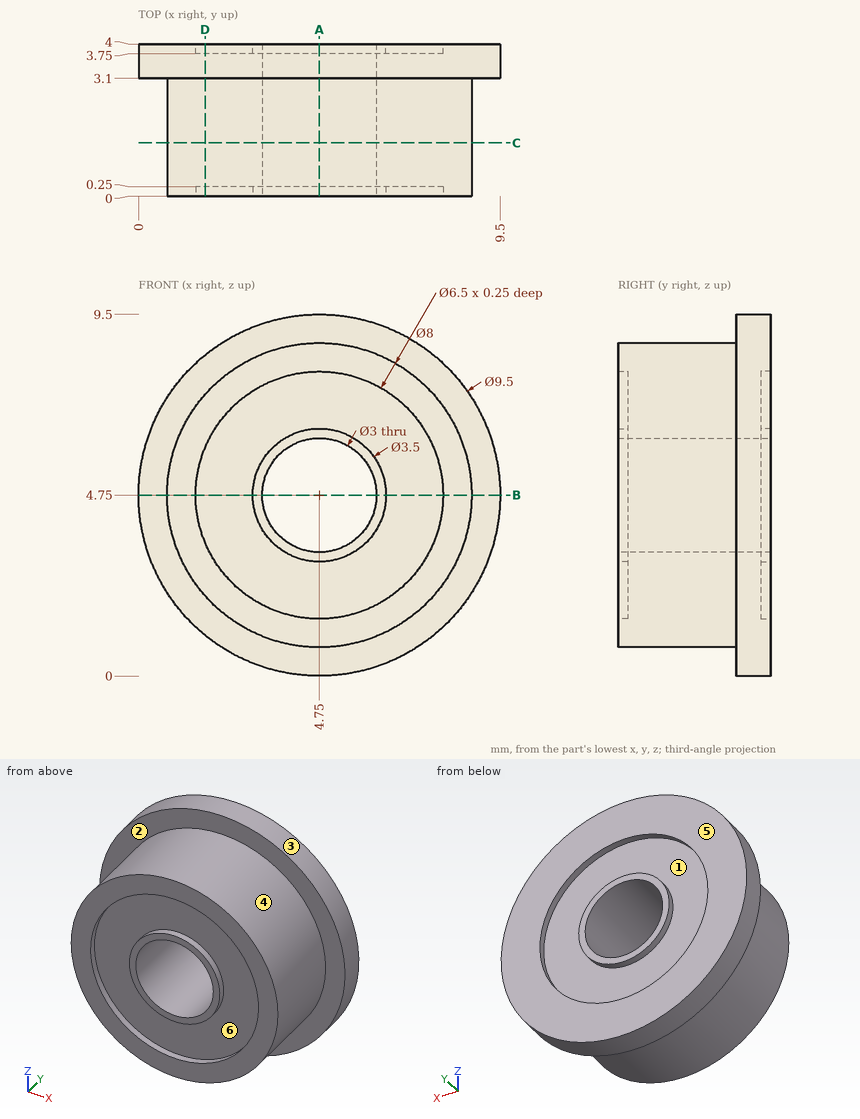
Print and shaded views of the part. All mm, measured from the part's lowest x, y and z. A direction names the side the tool comes from. Give positions to 0.01 mm unless a question says otherwise; leave off trailing zeros. Write each loop counter-clockwise with the first axis right and the second up, starting at its lowest first coordinate (ties: lowest second). Pieces come first, ordered by that corner, then holes. Notation, with made-up numbers: (36, -33.75) -> (62, -33.75) arc R24 ccw to (62, -20.75) -> close; hole circle Ø7 at (6.5, -30.75). An arc over 180 degrees is marked (long way). Use CSV: the item, a comma, the result in double quotes. Start each with the question number.
1) Cut at A-A on x = 4.75. List the corners of the cut face in (y, z), plus the area to 4 significant figures.
2) Drill centre lines: L1, parallel to X at y = 3.9, z = 4.75; L2, parallel to X at y = 0.15, z = 4.75; L3, parallel to X at y = 1.85, z = 4.75. Where is each one in solid material? Low to high.
3) Tool access for the marked faces 1, 2 and 3: list every direction of +Z, -Z, +X, -X, +Y, -Y with a clear straight run to the whole face (end or side of a thin tool).
4) Cut at D-D on x = 1.75. List the corners of the cut face in (y, z).
5) Cut at B-B on z = 4.75. List the corners of the cut face in (x, y), plus the area to 4 significant figures.
6) Cut at C-C on y = 1.4. List the corners of the cut face in (x, z).
7) Two-plate mould, pull along X, no slides. Class the marked faces 4, 5 and 6: released by +X, released by -X, zero draft, split by the parting line, or undercut.
8) Pin check, flat tips, straight feed: P1, Ø5, axis at x = 7.5, z = 5, coming from the -Y side; P2, Ø1.8, axis at x = 4.75, z = 4.75, coming from the -Y side. Stop position of each tip, or through.
Final values:
1,outline,"(0, 0.75) -> (3.1, 0.75) -> (3.1, 0) -> (4, 0) -> (4, 1.5) -> (3.75, 1.5) -> (3.75, 3) -> (4, 3) -> (4, 3.25) -> (0, 3.25) -> (0, 3) -> (0.25, 3) -> (0.25, 1.5) -> (0, 1.5) -> close; (0, 6.25) -> (4, 6.25) -> (4, 6.5) -> (3.75, 6.5) -> (3.75, 8) -> (4, 8) -> (4, 9.5) -> (3.1, 9.5) -> (3.1, 8.75) -> (0, 8.75) -> (0, 8) -> (0.25, 8) -> (0.25, 6.5) -> (0, 6.5) -> close"
1,area,"19.85 mm2"
2,L1,"x = 0 to 1.5, 3 to 3.25, 6.25 to 6.5, 8 to 9.5"
2,L2,"x = 0.75 to 1.5, 3 to 3.25, 6.25 to 6.5, 8 to 8.75"
2,L3,"x = 0.75 to 3.25, 6.25 to 8.75"
3,face 1,"+Y"
3,face 2,"-Y"
3,face 3,"+Y, -Y"
4,outline,"(0, 2.1) -> (3.1, 2.1) -> (3.1, 1.07) -> (4, 1.07) -> (4, 3.5) -> (3.75, 3.5) -> (3.75, 6) -> (4, 6) -> (4, 8.43) -> (3.1, 8.43) -> (3.1, 7.4) -> (0, 7.4) -> (0, 6) -> (0.25, 6) -> (0.25, 3.5) -> (0, 3.5) -> close"
5,outline,"(0, 3.1) -> (0.75, 3.1) -> (0.75, 0) -> (1.5, 0) -> (1.5, 0.25) -> (3, 0.25) -> (3, 0) -> (3.25, 0) -> (3.25, 4) -> (3, 4) -> (3, 3.75) -> (1.5, 3.75) -> (1.5, 4) -> (0, 4) -> close; (6.25, 0) -> (6.5, 0) -> (6.5, 0.25) -> (8, 0.25) -> (8, 0) -> (8.75, 0) -> (8.75, 3.1) -> (9.5, 3.1) -> (9.5, 4) -> (8, 4) -> (8, 3.75) -> (6.5, 3.75) -> (6.5, 4) -> (6.25, 4) -> close"
5,area,"19.85 mm2"
6,outline,"circle Ø8 at (4.75, 4.75); hole circle Ø3 at (4.75, 4.75)"
7,face 4,"split by the parting line"
7,face 5,"zero draft"
7,face 6,"undercut"
8,P1,"stops at y = 0"
8,P2,"passes through"
